Part print with two shaded views. Sizes in mm from the minimum x, y, z corner. A direction names the side the tool comes from. Give positions to 0.01 mm unless a question says otherwise; leave off trailing zeros. Order: outer loops, then holes, each group sorted by start corner. A loop starts at its lowest first (then second) coordinate and runs counter-clockwise, first axis right, second up. Notation, with made-up numbers: M 4.25,5 L 42.25,5 A31 cw 42.25,37 Z; hole C 77.5,46.25 d9. An arc over 180 degrees is marked long. Return JSON: item names as keys, results as strings. Group by question number.
1. Slice it at C-C on z = 2.65. Give the number of separate pieces and of enclosed holes in the cut face, then the cut area to 3 significant figures.
2. Slice it at B-B on x = 90.5. List the corners of the cut face in (y, z).
3. Slice it at A-A on x = 33. List the corners of the cut face in (y, z).
4. Slice it at D-D on y = 8. List the corners of the cut face in (x, z), then the cut area to 3 significant figures.
5. Wall check: probe 1 along Y at (x, z) = (83, 2.95); probe 2 along X at (y, z) = (25, 2.9) (1 decimal); probe 3 along X at (y, z) = (34.5, 2.95) (1 decimal). Give the ranges that are in metal, low to high. Write a range as [from, to].
6. Pin check, flat tips, straight feed: pin 1 (0.9 mm diameter, centred on x = 40, z = 1, fed in from -Y); pin 2 (5 mm diameter, centred on x = 47.5, y = 34.5, fed in from -Z). Stop position of each tip, or through.
7. 3-axis set-ups, long thin cutter, end or side, ignore diameter. For the marked faces 1 and 2: which of +Z, -Z, +X, -X, +Y, -Y reach the whole face in a straight line?
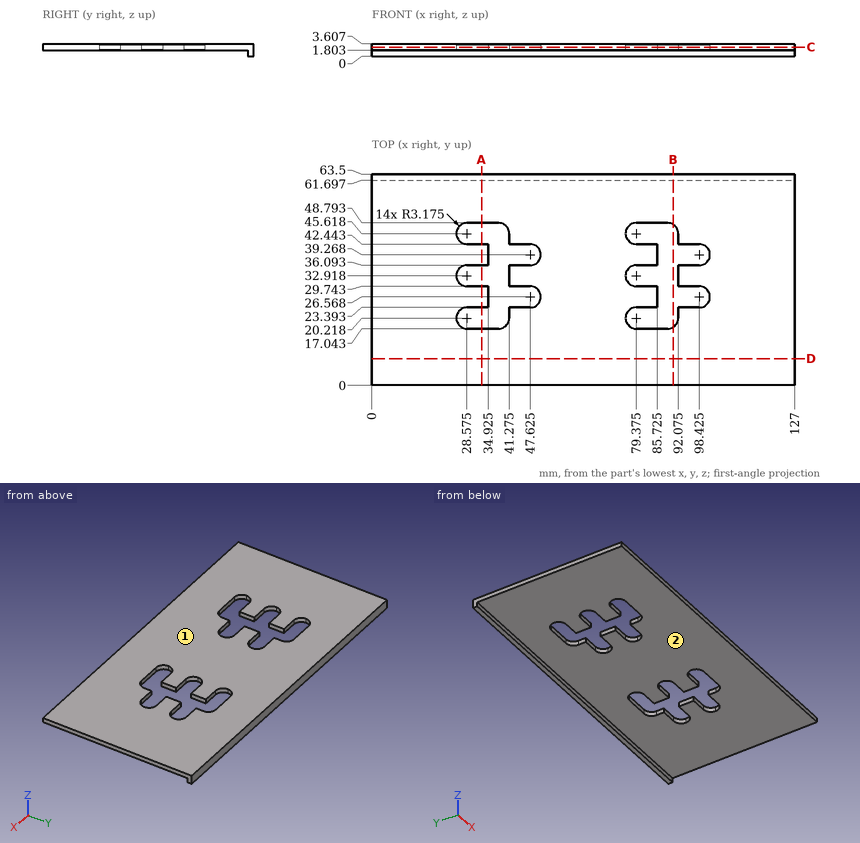
Result:
{
 "1": {"separate pieces": "1", "enclosed holes": "2", "area": "7,110 mm2"},
 "2": {"outline": "M 0,1.8 L 17.48,1.8 L 17.48,3.61 L 0,3.61 Z; M 48.36,1.8 L 61.7,1.8 L 61.7,0 L 63.5,0 L 63.5,3.61 L 48.36,3.61 Z"},
 "3": {"outline": "M 0,1.8 L 17.04,1.8 L 17.04,3.61 L 0,3.61 Z; M 23.39,1.8 L 29.74,1.8 L 29.74,3.61 L 23.39,3.61 Z; M 36.09,1.8 L 42.44,1.8 L 42.44,3.61 L 36.09,3.61 Z; M 48.79,1.8 L 61.7,1.8 L 61.7,0 L 63.5,0 L 63.5,3.61 L 48.79,3.61 Z"},
 "4": {"outline": "M 0,1.8 L 127,1.8 L 127,3.61 L 0,3.61 Z", "area": "229 mm2"},
 "5": {"probe 1": "y = [0, 17.04], [23.39, 29.74], [36.09, 42.44], [48.79, 63.5]", "probe 2": "x = [0, 34.9], [50.4, 85.7], [101.2, 127]", "probe 3": "x = [0, 25.8], [41.3, 76.6], [92.1, 127]"},
 "6": {"pin 1": "stops at y = 61.7", "pin 2": "stops at z = 1.8"},
 "7": {"face 1": "+Z, +X, -X, +Y, -Y", "face 2": "-Z, +X, -X, -Y"}
}
